Check sheet for the modelled part. Datum: model origin and axes. Units: mm. A direction names the side the tool comes from. Round coordinates to 2 decimals unless told otherwise and drop trailing zeros. Order: outer loops, then holes, each group sorted by start corner. A loop starts at its lowest first (then second) coordinate and runs counter-clockwise, first axis right, second up.
from build123d import *

# Parameters (mm, degrees)
SKETCH_1_R          = 42.5
EXTRUDE_1_DEPTH     = 10
SKETCH_2_R          = 39.5
CUT_EXTRUDE_1_DEPTH = 7
SKETCH_4_R          = 1.5
SKETCH_4_R_2        = 1.6
CUT_EXTRUDE_2_DEPTH = 61.930288035


with BuildPart() as part:
    # 草图1 → 凸台-拉伸1 (new body)
    with BuildSketch(Plane.XY):
        Circle(SKETCH_1_R)
    extrude(amount=EXTRUDE_1_DEPTH)

    # 草图2 → 切除-拉伸1 (cut)
    with BuildSketch(Plane(origin=(0, 0, 0), x_dir=(-1, 0, 0), z_dir=(0, 0, -1))):
        Circle(SKETCH_2_R)
    extrude(amount=-CUT_EXTRUDE_1_DEPTH, mode=Mode.SUBTRACT)

    # 草图4 → 切除-拉伸2 (cut, through all)
    with BuildSketch(Plane.XY.offset(10)):
        with Locations((0, 17.67766953)):
            Circle(SKETCH_4_R)
        with Locations((17.67766953, 0)):
            Circle(SKETCH_4_R)
        with Locations((0, -17.67766953)):
            Circle(SKETCH_4_R)
        with Locations((-17.67766953, 0)):
            Circle(SKETCH_4_R)
        Circle(SKETCH_4_R_2)
    extrude(amount=-CUT_EXTRUDE_2_DEPTH, mode=Mode.SUBTRACT)

    # 草图5 → 切除-旋转1 (revolve, cut)
    with BuildSketch(Plane(origin=(0, 0, 0), x_dir=(1, 0, 0), z_dir=(0, 1, 0)), mode=Mode.PRIVATE) as cut_revolve_1_sk:
        with BuildLine():
            Line((40.272743429, 0), (41.727256571, 0))
            ThreePointArc((41.727256571, 0), (41, -0.466686515), (40.272743429, 0))
        make_face()
    revolve(cut_revolve_1_sk.sketch.rotate(Axis((0, 0, -35.110243207), (0, 0, 1)), 180), axis=Axis((0, 0, -35.110243207), (0, 0, 1)), mode=Mode.SUBTRACT)


solid = part.part
1) Scan lines: line 1 (Y direction, x = 0, z = 8.55); line 2 (X direction, y = -0.5, z = 7.75); line 3 (Y direction, x = 0, z = 4). Record each from-to range of solid material in increasing order.
2) Gauge pin test, flat ends, axial feed: pin 1 (1 mm diameter, centred on y = 26.5, z = 8.5, fed in from -X); pin 2 (4 mm diameter, centred on x = -17.68, y = 0, fed in from -Z); pin 3 (4 mm diameter, centred on y = -16.5, z = 4, fed in from +X). Record the tip position at first contact, or that the pin passes through.
3) Sectioned sample at C-C on z = 1.5. Record the cut outline in (x, y), and give its area (3 significant figures).
4) Sectioned sample at A-A on y = 0. Record the cut outline in (x, z), and give its area (3 significant figures).
5) Set-up check for faces 4 (the face through (26.7, -29.6, 0)), 5 (the face through (29.11, 26.7, 3.45)): record each of +Z, -Z, +X, -X, +Y, -Y from which the full face is reachable in a straight line by a thin tool's end or side.
6) Draft check along Y on faces 1 (the face through (-19.176, 0.066, 8.521)), 2 (the face through (31.3, -28.1, 0)), 3 (the face through (-33.727, -25.861, 4.93)). Enter one of: pulls with the +Y half, pulls with the -Y half, needs draft (parallel to the pull), parting line crosses it, or undercut.
Values found:
1. line 1: y = -42.5 to -19.18, -16.18 to -1.6, 1.6 to 16.18, 19.18 to 42.5
1. line 2: x = -42.5 to -19.09, -16.26 to -1.52, 1.52 to 16.26, 19.09 to 42.5
1. line 3: y = -42.5 to -39.5, 39.5 to 42.5
2. pin 1: stops at x = -33.62
2. pin 2: stops at z = 7
2. pin 3: stops at x = 39.95
3. outline: circle Ø85 at (0, 0); hole circle Ø79 at (0, 0)
3. area: 773 mm2
4. outline: (-42.5, 0) - (-41.73, 0) arc R0.8 cw to (-40.27, 0) - (-39.5, 0) - (-39.5, 7) - (-19.18, 7) - (-19.18, 10) - (-42.5, 10) - close; (-16.18, 7) - (-1.6, 7) - (-1.6, 10) - (-16.18, 10) - close; (1.6, 7) - (16.18, 7) - (16.18, 10) - (1.6, 10) - close; (19.18, 7) - (39.5, 7) - (39.5, 0) - (40.27, 0) arc R0.8 cw to (41.73, 0) - (42.5, 0) - (42.5, 10) - (19.18, 10) - close
4. area: 268 mm2
5. face 4: -Z, +X, -X, +Y, -Y
5. face 5: -Z
6. face 1: undercut
6. face 2: needs draft
6. face 3: parting line crosses it
